```python
from build123d import *

# Parameters (mm, degrees)
SKETCH2_R           = 2.98
BOSS_EXTRUDE1_DEPTH = 20
FILLET1_R           = 6
FILLET2_R           = 2


with BuildPart() as part:
    # Sketch2 → Boss-Extrude1 (new, symmetric)
    with BuildSketch(Plane.XY):
        with BuildLine():
            Line((-6, 6), (6, 6))
            Line((6, 6), (6, -23.237900077))
            ThreePointArc((6, -23.237900077), (16.893008204, -17.047764481), (23.182219831, -6.211657082))
            Line((23.182219831, -6.211657082), (30.909626441, -8.282209443))
            ThreePointArc((30.909626441, -8.282209443), (19.480365728, -25.387306889), (0, -32))
            Line((0, -32), (-6, -32))
            Line((-6, -32), (-6, 6))
        make_face()
        Circle(SKETCH2_R, mode=Mode.SUBTRACT)
    extrude(amount=BOSS_EXTRUDE1_DEPTH, both=True)

    # Fillet1
    fillet1_edges = [part.edges().sort_by_distance(p)[0] for p in [
        (6, 6, 0),
        (-6, 6, 0),
        (-6, -32, 0),
    ]]
    fillet(fillet1_edges, radius=FILLET1_R - 0.0001)  # a hair under: the kernel refuses the full size

    # Fillet2
    fillet2_edges = [part.edges().sort_by_distance(p)[0] for p in [
        (6, -23.237900077, 0),
        (23.182219831, -6.211657082, 0),
        (30.909626441, -8.282209443, 0),
    ]]
    fillet(fillet2_edges, radius=FILLET2_R)


solid = part.part
```
Source: CAD feature listing. Evaluate the final solid. Frame: model axes, mm. A direction names the side the tool comes from. Give positions to 0.01 mm unless a question says otherwise; leave off trailing zeros. Loops run counter-clockwise (first coordinate to the right, second up) from the corner with the lowest first, then second, coordinate; pieces in that order, holes last. Notation, with made-up numbers: (-9.5, 16) - (27.5, 16) arc R22 ccw to (27.5, 28) - close; hole circle Ø10 at (6.5, -16.5). An arc over 180 degrees is marked (long way). Use CSV: the item, a comma, the result in double quotes.
1) Cut plane D-D (x = 7.5). Output: boundary loops of the cut face in (y, z), and give its area (3 significant figures).
Worked out:
outline,"(-31.11, -20) - (-22.43, -20) - (-22.43, 20) - (-31.11, 20) - close"
area,"347 mm^2"
2) Line query: line 1 (Y direction, x = 0, z = 3); line 2 (Y direction, x = 1, z = -10); line 3 (X direction, y = -1, z = 17). Output: solid intervals per line, ascending.
Worked out:
line 1,"y = -32 to -2.98, 2.98 to 6"
line 2,"y = -31.98 to -2.81, 2.81 to 5.92"
line 3,"x = -6 to -2.81, 2.81 to 6"
3) Cut plane C-C (y = -18). Output: boundary loops of the cut face in (x, z), and give its area (3 significant figures).
Worked out:
outline,"(-6, -20) - (6, -20) - (6, 20) - (-6, 20) - close; (15.87, -20) - (26.46, -20) - (26.46, 20) - (15.87, 20) - close"
area,"903 mm^2"
4) Cut plane B-B (x = -1.5). Output: boundary loops of the cut face in (y, z), and give its area (3 significant figures).
Worked out:
outline,"(-31.81, -20) - (-2.57, -20) - (-2.57, 20) - (-31.81, 20) - close; (2.57, -20) - (5.81, -20) - (5.81, 20) - (2.57, 20) - close"
area,"1,300 mm^2"
5) Set-up query: faces 1 (the flat face through (4, -17, -20)), 2 (the cylindrical face through (17.15, -16.79, 0.28)). Return all of +Z, -Z, +X, -X, +Y, -Y with unobstructed straight access to the full face (end or side cutting, diameter ignored); none if empty.
Worked out:
face 1,"-Z, +X, -X, +Y, -Y"
face 2,"+Z, -Z, +Y"
6) Mould query, pull axis Y, two halves, no side actions, for faces 3 (the flat face through (6, -10, 0)), 4 (the cylindrical face through (4.196, 4.289, -0.28)), 5 (the cylindrical face through (-0.388, 2.955, -0.28)). Classes: +Y half, -Y half, draft (parallel to the pull), parting line (faces both ways), or undercut.
Worked out:
face 3,"draft"
face 4,"+Y half"
face 5,"undercut"
7) Pin query (flat end, axial travel): P1, Ø7.5, axis at x = 0, y = 0, coming from the +Z side; P2, Ø1, axis at x = 15, z = 15, coming from the -Y side; P3, Ø4, axis at x = 24.5, y = -4, coming from the +Z side; P4, Ø2, axis at x = 7, z = 3.5, coming from the -Y side. Return the tip coordinate at first contact, or that it passes through.
Worked out:
P1,"stops at z = 20"
P2,"stops at y = -28.53"
P3,"passes through"
P4,"stops at y = -31.43"
